```python
from build123d import *

# Parameters (mm, degrees)
EXTRUDE_1_DEPTH          = 34
SKETCH_2_W               = 16.6
SKETCH_2_H               = 7.2
EXTRUDE_2_DEPTH          = 18
CUT_EXTRUDE_2_DEPTH      = 2.2
CHAMFER_1_SIZE           = 0.6
EXTRUDE_4_DEPTH          = 2
SKETCH_8_R               = 1.6
EXTRUDE_5_DEPTH          = 6
CUT_EXTRUDE_4_DEPTH      = 6
SKETCH_9_R               = 1
CUT_EXTRUDE_5_DEPTH      = 7
CUT_EXTRUDE_5_DEPTH_BACK = 4
SKETCH_10_R              = 1.65
CUT_EXTRUDE_6_DEPTH      = 6
FILLET_1_R               = 2
SKETCH_13_R              = 0.75
CUT_EXTRUDE_9_DEPTH      = 8.2
FILLET_2_R               = 2
CHAMFER_2_SIZE           = 1


with BuildPart() as part:
    # Sketch 1 → Extrude 1 (new body)
    with BuildSketch(Plane(origin=(0, 0, 0), x_dir=(1, 0, 0), z_dir=(0, 1, 0))):
        Polygon((-6.5, 0), (6.5, 0), (6.5, 6), (8.3, 6), (8.3, -1.2), (-8.3, -1.2), (-8.3, 6), (-6.5, 6), align=None)
    extrude(amount=EXTRUDE_1_DEPTH)

    # Sketch 2 → Extrude 2 (add)
    with BuildSketch(Plane(origin=(0, 34, 0), x_dir=(1, 0, 0), z_dir=(0, 1, 0))):
        with Locations((0, 2.4)):
            Rectangle(SKETCH_2_W, SKETCH_2_H)
    extrude(amount=EXTRUDE_2_DEPTH)

    # Sketch 4 → Cut-Extrude 2 (cut, through all)
    with BuildSketch(Plane(origin=(0, 0, 0), x_dir=(-1, 0, 0), z_dir=(0, 0, -1))):
        with BuildLine():
            Line((0.9, 25.5), (0.9, 21.5))
            ThreePointArc((0.9, 21.5), (0, 20.6), (-0.9, 21.5))
            Line((-0.9, 21.5), (-0.9, 25.5))
            ThreePointArc((-0.9, 25.5), (0, 26.4), (0.9, 25.5))
        make_face()
    extrude(amount=-CUT_EXTRUDE_2_DEPTH, mode=Mode.SUBTRACT)

    # Chamfer 1
    chamfer_1_edges = [part.edges().sort_by_distance(p)[0] for p in [
        (0, 26.4, 1.2),
        (-0.9, 23.5, 1.2),
        (0, 20.6, 1.2),
        (0.9, 23.5, 1.2),
    ]]
    chamfer(chamfer_1_edges, length=CHAMFER_1_SIZE)

    # Sketch 5 → Extrude 4 (add, symmetric)
    with BuildSketch(Plane(origin=(0, 23.5, 0), x_dir=(-1, 0, 0), z_dir=(0, -1, 0))):
        Polygon((-6.5, 6), (-4.15, 6), (-4.15, 0.6), (-2.15, 0.6), (-2.15, 0), (-6.5, 0), align=None)
        Polygon((6.5, 0), (6.5, 6), (4.15, 6), (4.15, 0.6), (2.15, 0.6), (2.15, 0), align=None)
    extrude(amount=EXTRUDE_4_DEPTH, both=True)

    # Sketch 8 → Extrude 5 (add)
    with BuildSketch(Plane(origin=(0, 0, -6), x_dir=(-1, 0, 0), z_dir=(0, 0, -1))):
        with BuildLine():
            Line((-5.5, 5), (-8.3, 5))
            Line((-8.3, 5), (-8.3, 0))
            Line((-8.3, 0), (-5.5, 0))
            ThreePointArc((-5.5, 0), (-3, 2.5), (-5.5, 5))
        make_face()
        with Locations((-5.5, 2.5)):
            Circle(SKETCH_8_R, mode=Mode.SUBTRACT)
        with BuildLine():
            Line((8.3, 0), (5.5, 0))
            ThreePointArc((5.5, 0), (3, 2.5), (5.5, 5))
            Line((5.5, 5), (8.3, 5))
            Line((8.3, 5), (8.3, 0))
        make_face()
        with Locations((5.5, 2.5)):
            Circle(SKETCH_8_R, mode=Mode.SUBTRACT)
    extrude(amount=-EXTRUDE_5_DEPTH)

    # Sketch 8_2 → Cut-Extrude 4 (cut)
    with BuildSketch(Plane(origin=(0, 0, -6), x_dir=(-1, 0, 0), z_dir=(0, 0, -1))):
        with BuildLine():
            Line((-6.5, 1.2510004), (-6.5, 3.7489996))
            ThreePointArc((-6.5, 3.7489996), (-7.1, 2.5), (-6.5, 1.2510004))
        make_face()
        with BuildLine():
            ThreePointArc((-3.9, 2.5), (-4.807179677, 3.94222051), (-6.5, 3.7489996))
            Line((-6.5, 3.7489996), (-6.5, 1.2510004))
            ThreePointArc((-6.5, 1.2510004), (-4.807179677, 1.05777949), (-3.9, 2.5))
        make_face()
        with BuildLine():
            Line((6.5, 3.7489996), (6.5, 1.2510004))
            ThreePointArc((6.5, 1.2510004), (6.94222051, 1.807179677), (7.1, 2.5))
            ThreePointArc((7.1, 2.5), (6.94222051, 3.192820323), (6.5, 3.7489996))
        make_face()
        with BuildLine():
            ThreePointArc((6.5, 3.7489996), (3.9, 2.5), (6.5, 1.2510004))
            Line((6.5, 1.2510004), (6.5, 3.7489996))
        make_face()
    extrude(amount=-CUT_EXTRUDE_4_DEPTH, mode=Mode.SUBTRACT)

    # Sketch 9 → Cut-Extrude 5 (cut, two sides)
    with BuildSketch(Plane(origin=(0, 0, 0), x_dir=(-1, 0, 0), z_dir=(0, 0, -1))) as cut_extrude_5_sk:
        with Locations(Location((-5.5, 2.5, 0), (0, 0, 180))):  # turned: the seam where the file's is
            Circle(SKETCH_9_R)
        with Locations(Location((5.5, 2.5, 0), (0, 0, 180))):  # turned: the seam where the file's is
            Circle(SKETCH_9_R)
        with Locations(Location((5.5, 48, 0), (0, 0, 180))):  # turned: the seam where the file's is
            Circle(SKETCH_9_R)
        with Locations(Location((-5.5, 48, 0), (0, 0, 180))):  # turned: the seam where the file's is
            Circle(SKETCH_9_R)
    extrude(amount=CUT_EXTRUDE_5_DEPTH, mode=Mode.SUBTRACT)
    extrude(cut_extrude_5_sk.sketch, amount=-CUT_EXTRUDE_5_DEPTH_BACK, mode=Mode.SUBTRACT)

    # Sketch 10 → Cut-Extrude 6 (cut)
    with BuildSketch(Plane(origin=(0, 0, -6), x_dir=(-1, 0, 0), z_dir=(0, 0, -1))):
        with Locations((-5.5, 48)):
            Circle(SKETCH_10_R)
        with Locations((5.5, 48)):
            Circle(SKETCH_10_R)
    extrude(amount=-CUT_EXTRUDE_6_DEPTH, mode=Mode.SUBTRACT)

    # Fillet 1
    fillet_1_edges = [part.edges().sort_by_distance(p)[0] for p in [
        (-6.5, 34, -3),
        (6.5, 34, -3),
    ]]
    fillet(fillet_1_edges, radius=FILLET_1_R)

    # Sketch 13 → Cut-Extrude 9 (cut, through all)
    with BuildSketch(Plane(origin=(0, 0, -6), x_dir=(-1, 0, 0), z_dir=(0, 0, -1))):
        with Locations((0, 40.551155153)):
            Circle(SKETCH_13_R)
        with Locations((-1.75, 37.52006624)):
            Circle(SKETCH_13_R)
        with Locations((1.75, 37.52006624)):
            Circle(SKETCH_13_R)
    extrude(amount=-CUT_EXTRUDE_9_DEPTH, mode=Mode.SUBTRACT)

    # Fillet 2
    fillet_2_edges = [part.edges().sort_by_distance(p)[0] for p in [
        (-8.3, 52, -2.4),
        (8.3, 52, -2.4),
        (8.3, 0, -2.4),
        (-8.3, 0, -2.4),
    ]]
    fillet(fillet_2_edges, radius=FILLET_2_R)

    # Chamfer 2
    chamfer_2_edges = [part.edges().sort_by_distance(p)[0] for p in [
        (8.3, 26, 1.2),
        (0, 0, 1.2),
        (0, 52, 1.2),
        (-8.3, 26, 1.2),
        (-7.714213562, 51.414213562, 1.2),
        (7.714213562, 51.414213562, 1.2),
        (-7.714213562, 0.585786438, 1.2),
        (7.714213562, 0.585786438, 1.2),
    ]]
    chamfer(chamfer_2_edges, length=CHAMFER_2_SIZE)


solid = part.part
```
Geometry: final body of the model. Coordinates: model frame, mm. A direction names the side the tool comes from. Coordinates: 2 decimals unless noted, no trailing zeros. Order: outer loops, then holes, each group sorted by start corner. A loop starts at its lowest first (then second) coordinate and runs counter-clockwise, first axis right, second up.
Item 1: Section query D-D (y = 15). Output: boundary loops of the cut face in (x, z).
Answer:
outline: (-8.3, -6) - (-6.5, -6) - (-6.5, 0) - (6.5, 0) - (6.5, -6) - (8.3, -6) - (8.3, 0.2) - (7.3, 1.2) - (-7.3, 1.2) - (-8.3, 0.2) - close
Item 2: Draft query along Y for faces 3 (the face through (7.8, 25.7, 0.7)), 4 (the face through (0, 52, -3)), 5 (the face through (0, 26.4, 0.3)). Return one class per face: released by +Y, released by -Y, zero draft, split by the parting line, or undercut.
Answer:
face 3: zero draft
face 4: released by +Y
face 5: undercut
Item 3: Contact query for flat-ended pins moving along their axis: P1, Ø1, axis at x = -6, y = 2, coming from the -Z side; P2, Ø3, axis at x = 2.5, z = -2.5, coming from the -Y side; P3, Ø1, axis at x = 3.5, y = 24, coming from the -Z side. Output: stop coordinate, or through.
Answer:
P1: stops at z = 0
P2: stops at y = 0.5
P3: stops at z = -0.6
Item 4: Section query B-B (x = 0). Output: boundary loops of the cut face in (y, z).
Answer:
outline: (0, 0) - (20.6, 0) - (20.6, 0.6) - (20, 1.2) - (1, 1.2) - (0, 0.2) - close; (26.4, 0) - (34, 0) - (34, -6) - (39.8, -6) - (39.8, 1.2) - (27, 1.2) - (26.4, 0.6) - close; (41.3, -6) - (52, -6) - (52, 0.2) - (51, 1.2) - (41.3, 1.2) - close
Item 5: Section query A-A (y = 48). Output: boundary loops of the cut face in (x, z).
Answer:
outline: (-8.3, -6) - (-7.15, -6) - (-7.15, 0) - (-6.5, 0) - (-6.5, 1.2) - (-7.3, 1.2) - (-8.3, 0.2) - close; (-4.5, 0) - (-3.85, 0) - (-3.85, -6) - (3.85, -6) - (3.85, 0) - (4.5, 0) - (4.5, 1.2) - (-4.5, 1.2) - close; (6.5, 0) - (7.15, 0) - (7.15, -6) - (8.3, -6) - (8.3, 0.2) - (7.3, 1.2) - (6.5, 1.2) - close
Item 6: Section query C-C (y = 25). Output: boundary loops of the cut face in (x, z), then the cut area to 3 significant figures.
Answer:
outline: (-8.3, -6) - (-4.15, -6) - (-4.15, -0.6) - (-2.15, -0.6) - (-2.15, 0) - (-0.9, 0) - (-0.9, 0.6) - (-1.5, 1.2) - (-7.3, 1.2) - (-8.3, 0.2) - close; (0.9, 0) - (2.15, 0) - (2.15, -0.6) - (4.15, -0.6) - (4.15, -6) - (8.3, -6) - (8.3, 0.2) - (7.3, 1.2) - (1.5, 1.2) - (0.9, 0.6) - close
area: 68.6 mm2
Item 7: Access query for faces 1 (the face through (0.1, 51.5, 0.7)), 2 (the face through (-6, 5, -3)). Directions: +Z, -Z, +X, -X, +Y, -Y. A direction counts if a zero-diameter tool reaches every point of the face in a straight line with its end or side. Return the directions, or none.
Answer:
face 1: +Z, +X, -X, +Y
face 2: -Z
Item 8: Material intervals for line 1 along X through (y, z) = (25, -5); line 2 along Y through (x, z) = (-5.5, 0.75); line 3 along X through (y, z) = (2.5, 0.85), sorted ascending.
Answer:
line 1: x = -8.3 to -4.15, 4.15 to 8.3
line 2: y = 0.55 to 1.5, 3.5 to 47, 49 to 51.45
line 3: x = -7.65 to -6.5, -4.5 to 4.5, 6.5 to 7.65
